Here's how the part is built. I have some questions about the finished solid (model axes, mm). Face numbers are marked on the shaded views. A direction names the side the tool comes from. Coordinates: 2 decimals unless noted, no trailing zeros. Loops run counter-clockwise (first coordinate to the right, second up) from the corner with the lowest first, then second, coordinate; pieces in that order, holes last. Notation, with made-up numbers: (5, -32) -> (35, -32) arc R16 ccw to (35, -19) -> close; hole circle Ø11 at (-22.75, 17). An arc over 180 degrees is marked (long way). Answer as a JSON object with one key per item and string values. Group by question number.
1) If we mould it in two halves opening along Z, with no side actions, what happens to the marked faces 3, 4, 5 and 6? For each: +Z half, -Z half, draft (parallel to the pull), parting line (faces both ways), or undercut.
2) I'm going to push flat-ended pins straight in: pin 1 (1 mm diameter, centred on x = 9.5, y = -7, fed in from +Z); pin 2 (6 mm diameter, centred on x = 43, y = 36, fed in from +Z); pin 3 (5 mm diameter, centred on x = 39, y = 21.5, fed in from +Z). Where does each tip first touch, or does it pass through?
3) I want a section at A-A (z = 9). Write out the boundary of the cut face in (x, y).
4) I want a section at B-B (y = 44). Write out the boundary of the cut face in (x, z).
5) I need wall thicknesses on probe 1 along Z at (x, y) = (32.5, 39); probe 2 along Z at (x, y) = (5, -35); probe 3 along Z at (x, y) = (31.5, 28). Which ranges of each line are inside material? Lowest first, please. Write a range as [from, to].
6) I want a section at C-C (z = 31.5). Write out the boundary of the cut face in (x, y).
7) Which directions (+Z, -Z, +X, -X, +Y, -Y) give clear straight access to the entire face, cutting with the end or side of a thin tool? Please do the marked faces 1 and 2.
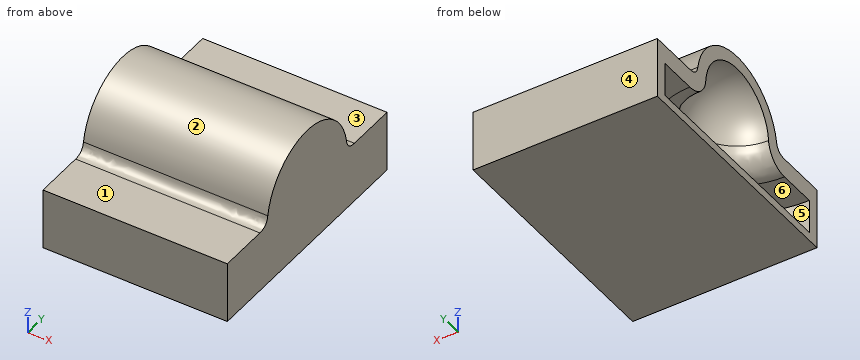
```python
from build123d import *

# Parameters (mm, degrees)
F1_DEPTH    = 76.2
F2_T1_DEPTH = 76.2
F5_R        = 10.16


# Not quite as in the source:
# - a fillet or chamfer that OpenCascade refuses, or shapes differently, is made with other operations: its cross-section is extruded or revolved along the edge and cut away or added


with BuildPart() as f1:
    # F0 (on Right) → F1 (new body)
    with BuildSketch(Plane.YZ):
        with BuildLine():
            Line((-50.8, 0), (0, 0))
            Line((0, 0), (50.8, 0))
            Line((50.8, 0), (50.8, 25.4))
            Line((50.8, 25.4), (25.4, 25.4))
            ThreePointArc((25.4, 25.4), (0, 50.8), (-25.4, 25.4))
            Line((-25.4, 25.4), (-50.8, 25.4))
            Line((-50.8, 25.4), (-50.8, 0))
        make_face()
    extrude(amount=F1_DEPTH)

    # F2: fillet of radius 5.08 on 2 edges, made by hand

    # F2_s2 → F2_t1 (join)
    with BuildSketch(Plane.YZ):
        with BuildLine():
            add(Edge.make_bspline(
                [(-30.0536852981, 25.4), (-25.7603016841, 25.4), (-25.0447377485, 29.6333333333)],
                knots=[0, 0, 0, 1, 1, 1], degree=2, weights=[1, 1, 1]))
            ThreePointArc((-25.0447377485, 29.6333333333), (-25.3110286122, 27.5241070111), (-25.4, 25.4))
            Line((-25.4, 25.4), (-30.0536852981, 25.4))
        make_face()
        with BuildLine():
            add(Edge.make_bspline(
                [(30.0536852981, 25.4), (25.7603016841, 25.4), (25.0447377485, 29.6333333333)],
                knots=[0, 0, 0, 1, 1, 1], degree=2, weights=[1, 1, 1]))
            ThreePointArc((25.0447377485, 29.6333333333), (25.3110286122, 27.5241070111), (25.4, 25.4))
            Line((25.4, 25.4), (30.0536852981, 25.4))
        make_face()
    extrude(amount=F2_T1_DEPTH)

    # F3 (on face) → F4 (revolve, cut)
    with BuildSketch(Plane(origin=(0, 0, 0), x_dir=(0, -1, 0), z_dir=(-1, 0, 0))):
        with BuildLine():
            Line((0, 45.441377908), (0, 3.5084052943))
            Line((0, 3.5084052943), (45.9408350289, 3.5084052943))
            Line((45.9408350289, 3.5084052943), (45.9408350289, 17.5937116146))
            Line((45.9408350289, 17.5937116146), (18.4585668484, 17.5937116146))
            ThreePointArc((18.4585668484, 17.5937116146), (16.7048736009, 36.4726702484), (0, 45.441377908))
        make_face()
    revolve(axis=Axis((0, 0, 24.4748916011), (0, 0, -1)), mode=Mode.SUBTRACT)

    # F5
    f5_edges = [f1.edges().sort_by_distance(p)[0] for p in [
        (18.458567, 0, 17.593712),
    ]]
    fillet(f5_edges, radius=F5_R)


solid = f1.part
```
Determined:
{
 "1": {"face 3": "+Z half", "face 4": "draft", "face 5": "undercut", "face 6": "undercut"},
 "2": {"pin 1": "z = 49.95", "pin 2": "z = 25.4", "pin 3": "z = 42.26"},
 "3": {"outline": "(0, -50.8) -> (76.2, -50.8) -> (76.2, 50.8) -> (0, 50.8) -> (0, 45.94) arc R45.94 cw to (0, -45.94) -> close"},
 "4": {"outline": "(0, 0) -> (76.2, 0) -> (76.2, 25.4) -> (0, 25.4) -> (0, 17.59) -> (13.21, 17.59) -> (13.21, 3.51) -> (0, 3.51) -> close"},
 "5": {"probe 1": "[0, 25.4]", "probe 2": "[0, 3.51], [17.59, 25.4]", "probe 3": "[0, 3.51], [17.59, 25.71]"},
 "6": {"outline": "(0, -24.66) -> (76.2, -24.66) -> (76.2, 24.66) -> (0, 24.66) -> (0, 19.09) arc R19.09 cw to (0, -19.09) -> close"},
 "7": {"face 1": "+Z, +X, -X, -Y", "face 2": "+Z, +X, -X"}
}
